Solid Edge part; units mm, degrees
sketch "Sketch1" plane through (0, 0, 0) normal (0, 0, 1) x (1, 0, 0)
  line L0 (0, 71.5) -> (0, 6.5)
  line L1 (13, 6.5) -> (13, 71.5)
  arc A0 (13, 6.5) -> (0, 6.5) centre (6.5, 6.5) cw
  arc A1 (0, 71.5) -> (13, 71.5) centre (6.5, 71.5) cw
extrude "Protrusion1" add sketch "Sketch1" along normal blind 6.5
sketch "Sketch2" plane through (6.5, 0, 0) normal (1, 0, 0) x (0, 1, 0)
  line L0 (3.5, 5.5) -> (3.5, 6.5)
  line L1 (3.5, 6.5) -> (6.5, 6.5)
  line L2 (6.5, 1) -> (6.5, 6.5)
  line L3 (3.5, 1) -> (6.5, 1)
  line L4 (3.5, 1) -> (2.6811, 3.25)
  line L5 (3.5, 5.5) -> (2.6811, 3.25)
revolve "RevolvedCutout1" cut sketch "Sketch2" angle 360 about axis through (6.5, 6.5, 1) along (0, 0, 1)
chamfer "Chaflán_38" distance 0.75 angle 45 1 edges at (6.5, 3.5, 6.5)
pattern_linear "Pattern1" count 6 spacing 13 along (0, 1, 0) of "RevolvedCutout1", "Chaflán_38"
chamfer "Chaflán_39" distance 1.5 angle 45 8 edges at (13, 39, 6.5) (6.5, 0, 6.5) (0, 39, 6.5) (6.5, 78, 6.5) (13, 39, 0) (6.5, 0, 0) (0, 39, 0) (6.5, 78, 0)
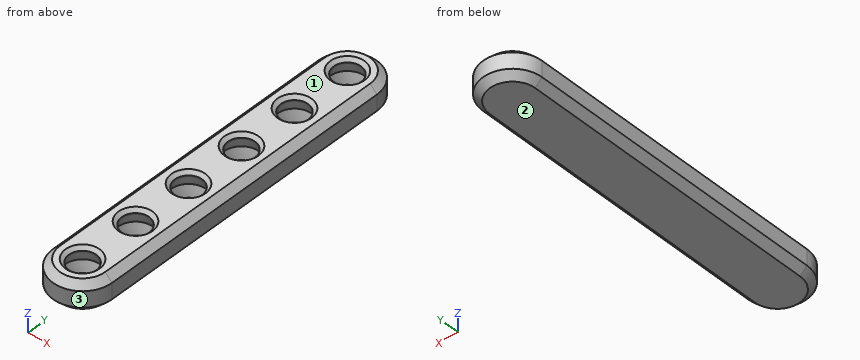
Design review of the part built by this model. Coordinates are the model's own, in mm. Face numbers are marked on the shaded views. Give positions to 0.01 mm unless a question says otherwise; leave off trailing zeros. Loops run counter-clockwise (first coordinate to the right, second up) from the corner with the lowest first, then second, coordinate; pieces in that order, holes last. Notation, with made-up numbers: (-7, -19) - (46, -19) arc R18 ccw to (46, -14) - close; hole circle Ø2 at (71, 77.5). An arc over 180 degrees is marked (long way). Write item = value, one per line.
1) Draft analysis for pull direction Z (two halves, no side actions). For the marked faces 1, 2 and 3, state which applies: +Z half, -Z half, draft (parallel to the pull), parting line (faces both ways), or undercut.
Result sheet:
face_1 = +Z half
face_2 = -Z half
face_3 = draft
2) Clearance check with flat-ended pins moving along their axes: pin 1 Ø1.8 at (x, y) = (6, 21) entering from +Z; pin 2 Ø3 at (x, z) = (4.5, 4.5) entering from -Y. State where each tip first meets the part, or that it passes through.
Result sheet:
pin_1 = 1
pin_2 = 0.02
3) To check wall thickness, follow line 1 (Z direction, x = 7, y = 6); line 2 (X direction, y = 18, z = 3.25); line 3 (X direction, y = 58.5, z = 5.75). State the ranges of each line that lie inside material, in increasing order.
Result sheet:
line_1 = 0 to 1
line_2 = 0 to 2.99, 10.01 to 13
line_3 = 0.75 to 3.5, 9.5 to 12.25
4) Take a section at A-A on y = 26.5. State the section outline as (x, z) points, and give its area (3 significant figures).
Result sheet:
outline = (0, 1.5) - (1.5, 0) - (11.5, 0) - (13, 1.5) - (13, 5) - (11.5, 6.5) - (1.5, 6.5) - (0, 5) - close
area = 80.0 mm2
5) Take a section at B-B on z = 4.25. State the section outline as (x, y) points, and give its area (3 significant figures).
Result sheet:
outline = (0, 6.5) arc R6.5 ccw to (13, 6.5) - (13, 71.5) arc R6.5 ccw to (0, 71.5) - close; hole circle Ø6.91 at (6.5, 6.5); hole circle Ø6.91 at (6.5, 19.5); hole circle Ø6.91 at (6.5, 32.5); hole circle Ø6.91 at (6.5, 45.5); hole circle Ø6.91 at (6.5, 58.5); hole circle Ø6.91 at (6.5, 71.5)
area = 753 mm2
